Solid Edge part; units mm, degrees
sketch "Sketch1" plane through (0, 0, 0) normal (0, -1, 0) x (1, 0, 0)
  line L0 (-20, 0) -> (-30, 60)
  line L1 (-30, 60) -> (-30, 80)
  line L2 (-30, 80) -> (30, 80)
  line L3 (30, 80) -> (30, 60)
  line L4 (30, 60) -> (20, 0)
  line L5 (20, 0) -> (-20, 0)
extrude "Protrusion1" add sketch "Sketch1" along normal blind 50
sketch "Sketch2" plane through (0, 0, 0) normal (0, -1, 0) x (1, 0, 0)
  circle A0 centre (0, 15) radius 7.5
extrude "Cutout1" cut sketch "Sketch2" along normal through all
sketch "Sketch3" plane through (0, 0, 0) normal (0, -1, 0) x (1, 0, 0)
  circle A0 centre (-15, 70) radius 5
extrude "Cutout2" cut sketch "Sketch3" along normal through all
sketch "Sketch4" plane through (0, 0, 0) normal (0, -1, 0) x (1, 0, 0)
  circle A0 centre (15, 70) radius 5
extrude "Cutout3" cut sketch "Sketch4" along normal through all
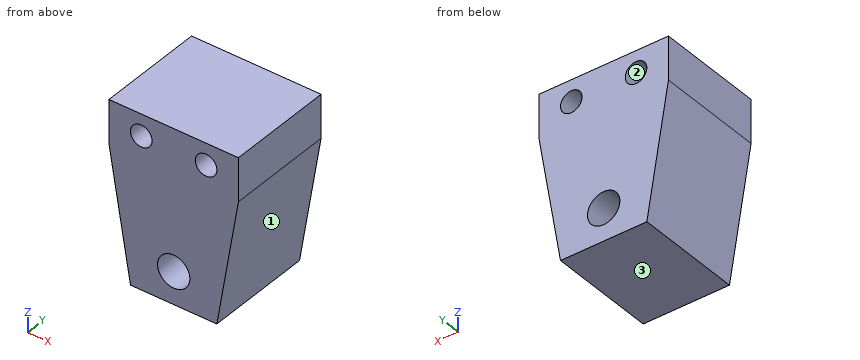
Model file for the job. Use its own axes, mm. Face numbers are marked on the shaded views. Coordinates: 2 decimals unless noted, no trailing zeros. Order: outer loops, then holes, each group sorted by start corner. A loop starts at its lowest first (then second) coordinate and runs counter-clockwise, first axis right, second up. Notation, with made-up numbers: M 35.25,13.5 L 55.25,13.5 A26 ccw 55.25,47.5 Z; hole C 76,8.5 d10. An arc over 180 degrees is marked long. Return JSON: item names as keys, results as strings.
1. Saw through at B-B (z = 15). Give the cut face in (x, y), and give its area (3 significant figures).
Ans:
{"outline": "M -22.5,-50 L -7.5,-50 L -7.5,0 L -22.5,0 Z; M 7.5,-50 L 22.5,-50 L 22.5,0 L 7.5,0 Z", "area": "1,500 mm^2"}
2. Saw through at C-C (y = -31.5). Give the cut face in (x, z).
Ans:
{"outline": "M -30,60 L -20,0 L 20,0 L 30,60 L 30,80 L -30,80 Z; hole C -15,70 d10; hole C 0,15 d15; hole C 15,70 d10"}
3. Saw through at A-A (x = 15). Give the cut face in (y, z), and give its area (3 significant figures).
Ans:
{"outline": "M -50,0 L 0,0 L 0,65 L -50,65 Z; M -50,75 L 0,75 L 0,80 L -50,80 Z", "area": "3,500 mm^2"}
4. Pull direction X, two halves, no side cores. Call the marked faces 1, 2 and 3: +X half, -X half, draft (parallel to the pull), parting line (faces both ways), or undercut.
Ans:
{"face 1": "+X half", "face 2": "undercut", "face 3": "draft"}
5. Drill centre lines: probe 1 along X at (y, z) = (-28, 70); probe 2 along Z at (x, y) = (15, -22); probe 3 along X at (y, z) = (-5.5, 74). Where is each one in solid material? Low to high.
Ans:
{"probe 1": "-30 to -20, -10 to 10, 20 to 30", "probe 2": "0 to 65, 75 to 80", "probe 3": "-30 to -18, -12 to 12, 18 to 30"}
6. Saw through at D-D (z = 70). Give the cut face in (x, y), and give its area (3 significant figures).
Ans:
{"outline": "M -30,-50 L -20,-50 L -20,0 L -30,0 Z; M -10,-50 L 10,-50 L 10,0 L -10,0 Z; M 20,-50 L 30,-50 L 30,0 L 20,0 Z", "area": "2,000 mm^2"}
7. Flat gauge pin, fed straight in: pin 1 (6 mm diameter, centred on x = 13, z = 32, fed in from +Y). Where does the tip first touch, or does it go through?
Ans:
{"pin 1": "y = 0"}
